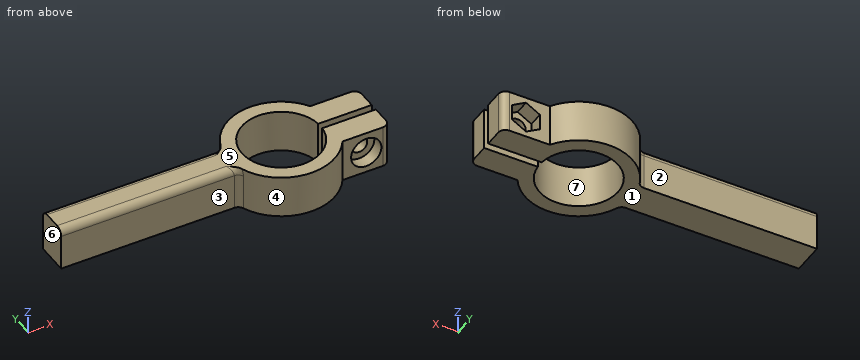
Autodesk Inventor part; units mm, degrees
ref_plane "YZ Plane" through (0, 0, 0) normal (1, 0, 0) x (0, 1, 0)
ref_plane "XZ Plane" through (0, 0, 0) normal (0, 1, 0) x (-1, 0, 0)
ref_plane "XY Plane" through (0, 0, 0) normal (0, 0, 1) x (1, 0, 0)
sketch "Sketch1" plane through (0, 0, 0) normal (0, 0, 1) x (1, 0, 0)
  circle A0 centre (0, 0) radius 11
  circle A1 centre (0, 0) radius 15
  line L0 (26, 8) -> (11, 8)
  line L1 (11, 8) -> (11, -8)
  line L2 (11, -8) -> (26, -8)
  line L3 (26, -8) -> (26, 8)
  line L4 (-64.309, 4.5) -> (-12, 4.5)
  line L5 (-12, 4.5) -> (-12, -4.5)
  line L6 (-12, -4.5) -> (-64.309, -4.5)
  line L7 (-64.309, -4.5) -> (-64.309, 4.5)
  point P0 (12.6886, 8)
  point P1 (12.6886, -8)
  point P2 (-14.3091, -4.5)
  point P3 (-14.3091, 4.5)
  dimension "d0" = 22
  dimension "d1" = 30
  dimension "d10" = 15
  dimension "d11" = 16
  dimension "d45" = 52.309
  dimension "d46" = 9
extrude "Extrusion1" add sketch "Sketch1" along normal blind 12
sketch "Sketch2" plane through (0, 0, 12) normal (0, 0, 1) x (1, 0, 0)
  circle A0 centre (0, 0) radius 11
  line L0 (26, -8) -> (26, 8)
  line L1 (26, 0) -> (10.8, 0)
  line L2 (10.8, 0) -> (10.8, 1)
  line L3 (10.8, 1) -> (26, 1)
  line L4 (26, 1) -> (26, 0)
  line L5 (26, 0) -> (10.8, 0)
  line L6 (10.8, 0) -> (10.8, -1)
  line L7 (10.8, -1) -> (26, -1)
  line L8 (26, -1) -> (26, 0)
  point P0 (10.9545, 1)
  point P1 (10.9545, -1)
  dimension "d20" = 15.2
  dimension "d21" = 1
  dimension "d22" = 1
extrude "Extrusion2" cut sketch "Sketch2" against normal blind 12 contours L1 L2 L3 A0 | L1 L0 L7 A0 | A0 L3 L0 L1 | A0 L7 L6 L1
sketch "Sketch3" plane through (12.6886, -8, 0) normal (0, -1, 0) x (1, 0, 0)
  line L0 (0, 0) -> (0, 12)
  line L1 (0, 0) -> (6.6555, 0)
  line L2 (6.6555, 0) -> (6.6555, 6)
  line L3 (6.6555, 6) -> (0, 6)
  line L4 (0, 6) -> (0, 0)
  point P0 (-12.6886, 0)
  dimension "d25" = 6.6555
  dimension "d26" = 6
hole "Hole1" at (19.3441, -8, 6) direction (0, 1, 0) diameter 4.5 depth 12.5 counterbore diameter 8.5 counterbore depth 3.5
sketch "Sketch4" plane through (12.6886, 8, 0) normal (0, 1, 0) x (1, 0, 0)
  line L0 (13.3114, 0) -> (0, 0)
  line L1 (0, 0) -> (6.6555, 0)
  line L2 (6.6555, 0) -> (6.6555, -6)
  line L3 (6.6555, -6) -> (0, -6)
  line L4 (0, -6) -> (0, 0)
  line L5 (6.6555, -6) -> (6.6555, -10.5)
  line L6 (6.6555, -6) -> (11.1555, -6) construction
  line L7 (6.6555, -10.5) -> (2.7584, -8.25)
  line L8 (2.7584, -8.25) -> (2.7584, -3.75)
  line L9 (2.7584, -3.75) -> (6.6555, -1.5)
  line L10 (6.6555, -1.5) -> (10.5526, -3.75)
  line L11 (10.5526, -3.75) -> (10.5526, -8.25)
  line L12 (10.5526, -8.25) -> (6.6555, -10.5)
  point P0 (-12.6886, 0)
  dimension "d51" = 6.6555
  dimension "d52" = 6
  dimension "d53" = 4.5
  dimension "d54" = 90
extrude "Extrusion3" cut sketch "Sketch4" against normal blind 4.2 contours L10 L11 L12 L5 L2 | L2 L3 L8 L9 | L5 L7 L8 L3
fillet "Fillet1" radius 2 2 edges at (-39.309, 4.5, 12) (-39.309, -4.5, 12)
fillet "Fillet2" radius 2 4 edges at (-14.3091, -4.5, 5) (-14.4562, -4.0024, 11.3202) (-14.3091, 4.5, 5) (-14.4562, 4.0024, 11.3201)
fillet "Fillet3" radius 2 2 edges at (26, -8, 6) (26, 8, 6)
properties part number "Clasp"
Source: CAD feature listing. Evaluate the final solid. Frame: model axes, mm. Face numbers are marked on the shaded views. A direction names the side the tool comes from. Round coordinates to 2 decimals unless told otherwise and drop trailing zeros. Loops run counter-clockwise (first coordinate to the right, second up) from the corner with the lowest first, then second, coordinate; pieces in that order, holes last.
(1) Pull-direction query (X, two-part tool) for the marked faces 4, 5, 6 and 7; classes: +X half, -X half, draft (parallel to the pull), parting line (faces both ways), or undercut.
From the geometry:
face 4: parting line
face 5: draft
face 6: -X half
face 7: undercut
(2) Section query A-A (x = 0). Output: boundary loops of the cut face in (y, z).
From the geometry:
outline: (-15, 0) - (-11, 0) - (-11, 12) - (-15, 12) - close; (11, 0) - (15, 0) - (15, 12) - (11, 12) - close
(3) Section query B-B (z = 6). Give the number of separate pieces and of enclosed holes in the cut face, and give its area (3 significant figures).
From the geometry:
separate pieces: 3
enclosed holes: 0
area: 839 mm2
(4) Access query for the marked faces 1, 2 and 3. Directions: +Z, -Z, +X, -X, +Y, -Y. A direction counts if a zero-diameter tool reaches every point of the face in a straight line with its end or side. Return the directions, or none.
From the geometry:
face 1: -Z, +X, -X, +Y, -Y
face 2: +Z, -Z, -X, +Y
face 3: +Z, -Z, -X, -Y
(5) Section query D-D (y = 0). Output: boundary loops of the cut face in (x, z), and give its area (3 significant figures).
From the geometry:
outline: (-64.31, 0) - (-11, 0) - (-11, 12) - (-64.31, 12) - close
area: 640 mm2
(6) Section query C-C (y = 9). Output: boundary loops of the cut face in (x, z), and give its area (3 significant figures).
From the geometry:
outline: (-12, 0) - (-6.32, 0) - (-6.32, 12) - (-12, 12) - close; (6.32, 0) - (12, 0) - (12, 12) - (6.32, 12) - close
area: 136 mm2
(7) Material intervals for probe 1 along Y at (x, z) = (17.5, 9.25); probe 2 along X at (y, z) = (-7, 2.25); probe 3 along X at (y, z) = (-6, 2.25), sorted ascending.
From the geometry:
probe 1: y = -4.5 to -1, 1 to 3.8
probe 2: x = -13.27 to -8.49, 8.49 to 17.34, 21.34 to 25.73
probe 3: x = -13.75 to -9.22, 9.22 to 17.34, 21.34 to 26
(8) Contact query for flat-ended pins moving along their axis: pin 1 Ø2 at (x, z) = (-14.5, 4.5) entering from +Y; pin 2 Ø7 at (x, z) = (19.34, 6) entering from +Y; pin 3 Ø2.5 at (x, z) = (17.5, 8) entering from -Y. Output: stop coordinate, or through.
From the geometry:
pin 1: stops at y = 6.54
pin 2: stops at y = 3.8
pin 3: stops at y = -4.5
